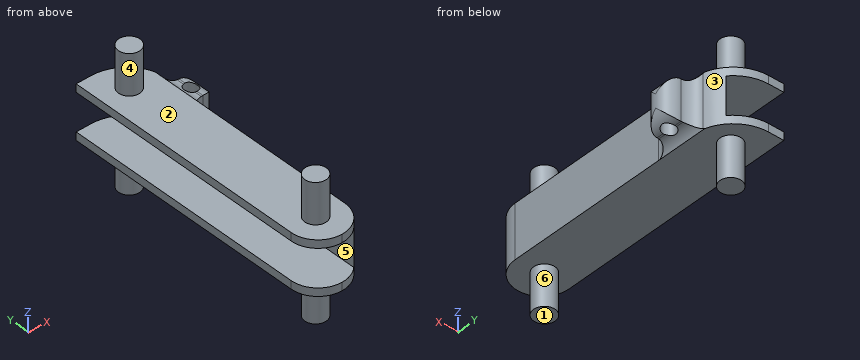
from build123d import *

# Parameters (mm, degrees)
SKETCH1_W               = 20
SKETCH1_H               = 100
BOSS_EXTRUDE1_DEPTH     = 10
SKETCH3_R               = 4
BOSS_EXTRUDE2_DEPTH     = 25
FILLET1_R               = 10
SKETCH5_W               = 10
SKETCH5_H               = 10
SKETCH5_R               = 2.5
BOSS_EXTRUDE3_DEPTH     = 7.5
FILLET2_R               = 5
CUT_EXTRUDE1_DEPTH      = 106.000000019
CUT_EXTRUDE1_DEPTH_BACK = 106.000000019
SKETCH6_W               = 17
SKETCH6_H               = 14
FILLET3_R               = 15


# Some blends are built 0.0001 mm under size
with BuildPart() as part:
    # Sketch1 → Boss-Extrude1 (new, symmetric)
    with BuildSketch(Plane(origin=(0, 0, 0), x_dir=(0, 0, -1), z_dir=(1, 0, 0))):
        with Locations((0, 50)):
            Rectangle(SKETCH1_W, SKETCH1_H)
    extrude(amount=BOSS_EXTRUDE1_DEPTH, both=True)

    # Sketch3 → Boss-Extrude2 (add, symmetric)
    with BuildSketch(Plane.XY):
        with Locations(Location((0, 11, 0), (0, 0, 270))):
            Circle(SKETCH3_R)
        with Locations(Location((0, 89, 0), (0, 0, 270))):
            Circle(SKETCH3_R)
    extrude(amount=BOSS_EXTRUDE2_DEPTH, both=True)

    # Fillet1
    fillet1_edges = [part.edges().sort_by_distance(p)[0] for p in [
        (10, 0, 0),
        (-10, 0, 0),
    ]]
    fillet(fillet1_edges, radius=FILLET1_R - 0.0001)  # a hair under: the kernel refuses the full size

    # Sketch5 → Boss-Extrude3 (add, symmetric)
    with BuildSketch(Plane.XY):
        with Locations((15, 80)):
            Rectangle(SKETCH5_W, SKETCH5_H)
        with Locations((15, 80)):
            Circle(SKETCH5_R, mode=Mode.SUBTRACT)
    extrude(amount=BOSS_EXTRUDE3_DEPTH, both=True)

    # Fillet2
    # the kernel refuses this fillet: 5 mm, written as the material it takes off along each edge
    with BuildSketch(Plane(origin=(20, 97.5, 7.5), x_dir=(-1, 0, 0), z_dir=(0, -1, 0))) as fillet2_piece_1:
        with BuildLine():
            CenterArc((FILLET2_R, FILLET2_R), FILLET2_R, 180, 90)
            Line((0, FILLET2_R), (0, 0))
            Line((0, 0), (FILLET2_R, 0))
        make_face()
    extrude(amount=35, mode=Mode.SUBTRACT)
    with BuildSketch(Plane(origin=(20, 97.5, -7.5), x_dir=(-1, 0, 0), z_dir=(0, -1, 0))) as fillet2_piece_2:
        with BuildLine():
            CenterArc((FILLET2_R, -FILLET2_R), FILLET2_R, 90, 90)
            Line((0, -FILLET2_R), (0, 0))
            Line((0, 0), (FILLET2_R, 0))
        make_face()
    extrude(amount=35, mode=Mode.SUBTRACT)
    with BuildSketch(Plane(origin=(20, 75, 20), x_dir=(-1, 0, 0), z_dir=(0, 0, -1))) as fillet2_piece_3:
        with BuildLine():
            CenterArc((FILLET2_R, FILLET2_R), FILLET2_R, 180, 90)
            Line((0, FILLET2_R), (0, 0))
            Line((0, 0), (FILLET2_R, 0))
        make_face()
    extrude(amount=40, mode=Mode.SUBTRACT)
    with BuildSketch(Plane(origin=(20, 85, 20), x_dir=(-1, 0, 0), z_dir=(0, 0, -1))) as fillet2_piece_4:
        with BuildLine():
            CenterArc((FILLET2_R, -FILLET2_R), FILLET2_R, 90, 90)
            Line((0, -FILLET2_R), (0, 0))
            Line((0, 0), (FILLET2_R, 0))
        make_face()
    extrude(amount=40, mode=Mode.SUBTRACT)
    # the kernel refuses this fillet: 5 mm, written as the material it adds along each edge
    with BuildSketch(Plane(origin=(10, 75, 7.5), x_dir=(0, 0, 1), z_dir=(0, 1, 0))) as fillet2_2_piece_1_section:
        with BuildLine():
            CenterArc((5, 4.330127019), FILLET2_R, 180, 60)
            Line((0, 4.330127019), (0, 0))
            Line((0, 0), (2.5, 0))
        make_face()
    fillet2_2_piece_1 = extrude(amount=10, mode=Mode.PRIVATE)
    fillet2_2_piece_1 = fillet2_2_piece_1 - Plane(origin=(15, 80, 7.5), x_dir=(1, 0, 0), z_dir=(0, 0, -1)) * Cylinder(2.5, 38, mode=Mode.PRIVATE)
    add(fillet2_2_piece_1)
    with BuildSketch(Plane(origin=(10, 75, -7.5), x_dir=(0, 0, -1), z_dir=(0, 1, 0))) as fillet2_2_piece_2_section:
        with BuildLine():
            CenterArc((5, -4.330127019), FILLET2_R, 120, 60)
            Line((0, -4.330127019), (0, 0))
            Line((0, 0), (2.5, 0))
        make_face()
    fillet2_2_piece_2 = extrude(amount=10, mode=Mode.PRIVATE)
    fillet2_2_piece_2 = fillet2_2_piece_2 - Plane(origin=(15, 80, -7.5), x_dir=(1, 0, 0), z_dir=(0, 0, -1)) * Cylinder(2.5, 38, mode=Mode.PRIVATE)
    add(fillet2_2_piece_2)
    with BuildSketch(Plane(origin=(10, 85, -7.5), x_dir=(0, 1, 0), z_dir=(0, 0, 1))) as fillet2_2_piece_3:
        with BuildLine():
            CenterArc((FILLET2_R, -FILLET2_R), FILLET2_R, 90, 90)
            Line((0, -FILLET2_R), (0, 0))
            Line((0, 0), (FILLET2_R, 0))
        make_face()
    extrude(amount=15)
    with BuildSketch(Plane(origin=(10, 75, -7.5), x_dir=(0, -1, 0), z_dir=(0, 0, 1))) as fillet2_2_piece_4:
        with BuildLine():
            CenterArc((FILLET2_R, FILLET2_R), FILLET2_R, 180, 90)
            Line((0, FILLET2_R), (0, 0))
            Line((0, 0), (FILLET2_R, 0))
        make_face()
    extrude(amount=15)
    with BuildSketch(Plane(origin=(10, 64.174682453, 7.5), x_dir=(0, 0, 1), z_dir=(0, 1, 0))) as fillet2_2_piece_5a_section:
        with BuildLine():
            CenterArc((5, 4.330127019), FILLET2_R, 180, 60)
            Line((0, 4.330127019), (0, 0))
            Line((0, 0), (2.5, 0))
        make_face()
    fillet2_2_piece_5a = extrude(amount=20.825317547, mode=Mode.PRIVATE)
    fillet2_2_piece_5a = split(fillet2_2_piece_5a, bisect_by=Plane(origin=(10, 75, 7.5), z_dir=(0, -1, 0)), keep=Keep.TOP, mode=Mode.PRIVATE)
    with BuildSketch(Plane(origin=(10, 75, -7.5), x_dir=(0, -1, 0), z_dir=(0, 0, 1))) as fillet2_2_piece_5b_section:
        with BuildLine():
            CenterArc((FILLET2_R, FILLET2_R), FILLET2_R, 180, 90)
            Line((0, FILLET2_R), (0, 0))
            Line((0, 0), (FILLET2_R, 0))
        make_face()
    fillet2_2_piece_5b = extrude(amount=27.5, mode=Mode.PRIVATE)
    fillet2_2_piece_5b = split(fillet2_2_piece_5b, bisect_by=Plane(origin=(10, 75, 10), z_dir=(0, 0, -1)), keep=Keep.TOP, mode=Mode.PRIVATE)
    fillet2_2_piece_5b = split(fillet2_2_piece_5b, bisect_by=Plane(origin=(10, 75, 7.5), z_dir=(0, 0, 1)), keep=Keep.TOP, mode=Mode.PRIVATE)
    fillet2_2_piece_5 = fillet2_2_piece_5a & fillet2_2_piece_5b
    add(fillet2_2_piece_5)
    with BuildSketch(Plane(origin=(10, 85, -7.5), x_dir=(0, 1, 0), z_dir=(0, 0, 1))) as fillet2_2_piece_6a_section:
        with BuildLine():
            CenterArc((FILLET2_R, -FILLET2_R), FILLET2_R, 90, 90)
            Line((0, -FILLET2_R), (0, 0))
            Line((0, 0), (FILLET2_R, 0))
        make_face()
    fillet2_2_piece_6a = extrude(amount=27.5, mode=Mode.PRIVATE)
    fillet2_2_piece_6a = split(fillet2_2_piece_6a, bisect_by=Plane(origin=(10, 85, 10), z_dir=(0, 0, -1)), keep=Keep.TOP, mode=Mode.PRIVATE)
    fillet2_2_piece_6a = split(fillet2_2_piece_6a, bisect_by=Plane(origin=(10, 85, 7.5), z_dir=(0, 0, 1)), keep=Keep.TOP, mode=Mode.PRIVATE)
    with BuildSketch(Plane(origin=(10, 75, 7.5), x_dir=(0, 0, 1), z_dir=(0, 1, 0))) as fillet2_2_piece_6b_section:
        with BuildLine():
            CenterArc((5, 4.330127019), FILLET2_R, 180, 60)
            Line((0, 4.330127019), (0, 0))
            Line((0, 0), (2.5, 0))
        make_face()
    fillet2_2_piece_6b = extrude(amount=20.825317547, mode=Mode.PRIVATE)
    fillet2_2_piece_6b = split(fillet2_2_piece_6b, bisect_by=Plane(origin=(10, 85, 7.5), z_dir=(0, 1, 0)), keep=Keep.TOP, mode=Mode.PRIVATE)
    fillet2_2_piece_6 = fillet2_2_piece_6a & fillet2_2_piece_6b
    add(fillet2_2_piece_6)
    with BuildSketch(Plane(origin=(10, 75, -20), x_dir=(0, -1, 0), z_dir=(0, 0, 1))) as fillet2_2_piece_7a_section:
        with BuildLine():
            CenterArc((FILLET2_R, FILLET2_R), FILLET2_R, 180, 90)
            Line((0, FILLET2_R), (0, 0))
            Line((0, 0), (FILLET2_R, 0))
        make_face()
    fillet2_2_piece_7a = extrude(amount=27.5, mode=Mode.PRIVATE)
    fillet2_2_piece_7a = split(fillet2_2_piece_7a, bisect_by=Plane(origin=(10, 75, -10), z_dir=(0, 0, 1)), keep=Keep.TOP, mode=Mode.PRIVATE)
    fillet2_2_piece_7a = split(fillet2_2_piece_7a, bisect_by=Plane(origin=(10, 75, -7.5), z_dir=(0, 0, -1)), keep=Keep.TOP, mode=Mode.PRIVATE)
    with BuildSketch(Plane(origin=(10, 64.174682453, -7.5), x_dir=(0, 0, -1), z_dir=(0, 1, 0))) as fillet2_2_piece_7b_section:
        with BuildLine():
            CenterArc((5, -4.330127019), FILLET2_R, 120, 60)
            Line((0, -4.330127019), (0, 0))
            Line((0, 0), (2.5, 0))
        make_face()
    fillet2_2_piece_7b = extrude(amount=20.825317547, mode=Mode.PRIVATE)
    fillet2_2_piece_7b = split(fillet2_2_piece_7b, bisect_by=Plane(origin=(10, 75, -7.5), z_dir=(0, -1, 0)), keep=Keep.TOP, mode=Mode.PRIVATE)
    fillet2_2_piece_7 = fillet2_2_piece_7a & fillet2_2_piece_7b
    add(fillet2_2_piece_7)
    with BuildSketch(Plane(origin=(10, 85, -20), x_dir=(0, 1, 0), z_dir=(0, 0, 1))) as fillet2_2_piece_8a_section:
        with BuildLine():
            CenterArc((FILLET2_R, -FILLET2_R), FILLET2_R, 90, 90)
            Line((0, -FILLET2_R), (0, 0))
            Line((0, 0), (FILLET2_R, 0))
        make_face()
    fillet2_2_piece_8a = extrude(amount=27.5, mode=Mode.PRIVATE)
    fillet2_2_piece_8a = split(fillet2_2_piece_8a, bisect_by=Plane(origin=(10, 85, -10), z_dir=(0, 0, 1)), keep=Keep.TOP, mode=Mode.PRIVATE)
    fillet2_2_piece_8a = split(fillet2_2_piece_8a, bisect_by=Plane(origin=(10, 85, -7.5), z_dir=(0, 0, -1)), keep=Keep.TOP, mode=Mode.PRIVATE)
    with BuildSketch(Plane(origin=(10, 75, -7.5), x_dir=(0, 0, -1), z_dir=(0, 1, 0))) as fillet2_2_piece_8b_section:
        with BuildLine():
            CenterArc((5, -4.330127019), FILLET2_R, 120, 60)
            Line((0, -4.330127019), (0, 0))
            Line((0, 0), (2.5, 0))
        make_face()
    fillet2_2_piece_8b = extrude(amount=20.825317547, mode=Mode.PRIVATE)
    fillet2_2_piece_8b = split(fillet2_2_piece_8b, bisect_by=Plane(origin=(10, 85, -7.5), z_dir=(0, 1, 0)), keep=Keep.TOP, mode=Mode.PRIVATE)
    fillet2_2_piece_8 = fillet2_2_piece_8a & fillet2_2_piece_8b
    add(fillet2_2_piece_8)

    # Sketch6 → Cut-Extrude1 (cut, two sides: drawn at the far end of the back side and taken through both)
    with BuildSketch(Plane(origin=(0, 100, 0), x_dir=(1, 0, 0), z_dir=(0, 1, 0)).offset(-CUT_EXTRUDE1_DEPTH_BACK)):
        with Locations((-1.5, 0)):
            Rectangle(SKETCH6_W, SKETCH6_H)
    extrude(amount=CUT_EXTRUDE1_DEPTH + CUT_EXTRUDE1_DEPTH_BACK, mode=Mode.SUBTRACT)

    # Fillet3
    # the kernel refuses this fillet: 15 mm, written as the material it takes off along each edge
    with BuildSketch(Plane(origin=(10, 100, -45.912291828), x_dir=(0.014111556263048879, -0.9999004270325296, 0), z_dir=(0, 0, 1))) as fillet3_piece_1:
        with BuildLine():
            CenterArc((14.795795075, -14.575159718), FILLET3_R, 103.668952733, 75.522487814)
            Line((-0.202711331, -14.363486374), (-1.702561971, -14.342319039))
            Line((-1.702561971, -14.342319039), (-1.499850641, 0.021167334))
            Line((-1.499850641, 0.021167334), (0.021167334, 1.499850641))
            ThreePointArc((0.021167334, 1.499850641), (10.020171605, 1.358735078), (10.896652831, 1.457515972))
            Line((10.896652831, 1.457515972), (11.251120307, 0))
        make_face()
    extrude(amount=91.824583655, mode=Mode.SUBTRACT)


solid = part.part
For this review, take the finished solid that the model builds, in its own axes (mm). Face numbers are marked on the shaded views. A direction names the side the tool comes from. Round coordinates to 2 decimals unless told otherwise and drop trailing zeros. Order: outer loops, then holes, each group sorted by start corner. A loop starts at its lowest first (then second) coordinate and runs counter-clockwise, first axis right, second up. Notation, with made-up numbers: (-39.5, -14) -> (-15.5, -14) arc R8 cw to (-15.5, -7) -> close; hole circle Ø6 at (12, 7). An arc over 180 degrees is marked (long way). Write item = value, one per line. Start each with the question number.
1) Take a section at C-C on y = 80. State the section outline as (x, z) points.
2) Insertion check: pin 1 (0.7 mm diameter, centred on x = 15, y = 84.5, fed in from -Z); pin 2 (10 mm diameter, centred on x = 0.5, y = 69.5, fed in from +Z); pin 3 (1 mm diameter, centred on y = 54.5, z = -6.5, fed in from +X); pin 4 (12 mm diameter, centred on y = 75, z = 19, fed in from -X). Each pin has a flat end and moves straight along its axis. Give the tip position at first contact, or say it passes through.
3) The part is to be moulded in two halves that separate along Y. For the marked faces 1, 2 and 3, say which applies: +Y half, -Y half, draft (parallel to the pull), parting line (faces both ways), or undercut.
4) To check wall thickness, follow line 1 (X direction, y = 80, z = -0.5); line 2 (Y direction, x = 15, z = 3); line 3 (Z direction, x = -1.5, y = 80). State the ranges of each line that lie inside material, in increasing order. Write a range as from..to.
5) Tool access review of the marked faces 4, 5 and 6: name each direction out of +Z, -Z, +X, -X, +Y, -Y from which nothing blocks a thin tool from reaching the whole face with its end or side.
6) Take a section at D-D on z = -19.5. State the section outline as (x, y) points.
7) Take a section at A-A on y = 11. State the section outline as (x, z) points, plus the area to 3 significant figures.
8) Take a section at B-B on x = 5. State the section outline as (y, z) points, plus the area to 3 significant figures.
Verdict:
q1.outline = (-10, -10) -> (10, -10) arc R5 cw to (12.5, -7.85) -> (12.5, 7.85) arc R5 cw to (10, 10) -> (-10, 10) -> (-10, 7) -> (7, 7) -> (7, -7) -> (-10, -7) -> close; (17.5, -6.83) arc R5 ccw to (20, -2.5) -> (20, 2.5) arc R5 ccw to (17.5, 6.83) -> close
q2.pin_1 = -7.5
q2.pin_2 = 10
q2.pin_3 = 10
q2.pin_4 = through
q3.face_1 = draft
q3.face_2 = undercut
q3.face_3 = +Y half
q4.line_1 = 7..12.5, 17.5..20
q4.line_2 = 75..77.5, 82.5..85
q4.line_3 = -10..-7, 7..10
q5.face_4 = +Z
q5.face_5 = -X, +Y, -Y
q5.face_6 = -Z
q6.outline = circle Ø8 at (0, 11); circle Ø8 at (0, 89)
q7.outline = (-10, -10) -> (-4, -10) -> (-4, -25) -> (4, -25) -> (4, -10) -> (10, -10) -> (10, 10) -> (4, 10) -> (4, 25) -> (-4, 25) -> (-4, 10) -> (-10, 10) -> (-10, 7) -> (7, 7) -> (7, -7) -> (-10, -7) -> close
q7.area = 402 mm2
q8.outline = (1.34, -10) -> (96.72, -10) -> (96.72, -7) -> (1.34, -7) -> close; (1.34, 7) -> (96.72, 7) -> (96.72, 10) -> (1.34, 10) -> close
q8.area = 572 mm2
